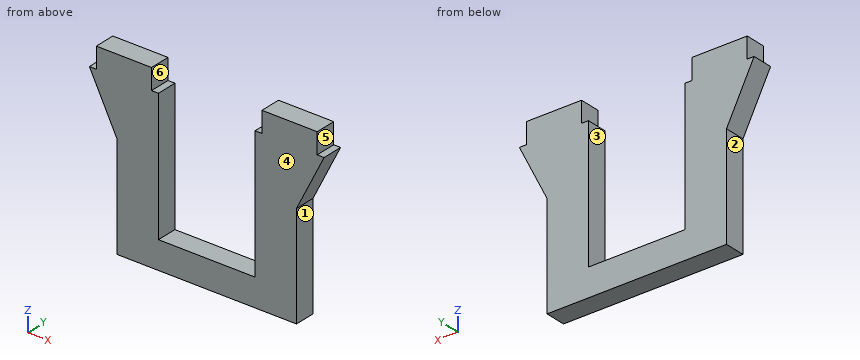
```python
from build123d import *

# Parameters (mm, degrees)
BOSS_EXTRUDE1_DEPTH = 1.5
BOSS_EXTRUDE2_DEPTH = 1.5
SKETCH3_W           = 8
SKETCH3_H           = 3
BOSS_EXTRUDE3_DEPTH = 1.5


with BuildPart() as part:
    # Sketch1 → Boss-Extrude1 (new body, symmetric)
    with BuildSketch(Plane(origin=(0, 0, 0), x_dir=(1, 0, 0), z_dir=(0, 1, 0))):
        Polygon((7, -9.5), (13, -9.5), (13, 13.5), (-13, 13.5), (-13, -9.5), (-7, -9.5), (-7, 9.5), (7, 9.5), align=None)
    extrude(amount=BOSS_EXTRUDE1_DEPTH, both=True)

    # Sketch2 → Boss-Extrude2 (add, symmetric)
    with BuildSketch(Plane(origin=(0, 0, 0), x_dir=(1, 0, 0), z_dir=(0, 1, 0))):
        Polygon((-13, -1.5), (-17, -9.5), (-13, -9.5), align=None)
        Polygon((13, -9.5), (13, -1.5), (17, -9.5), align=None)
    extrude(amount=BOSS_EXTRUDE2_DEPTH, both=True)

    # Sketch3 → Boss-Extrude3 (add, symmetric)
    with BuildSketch(Plane(origin=(0, 0, 0), x_dir=(1, 0, 0), z_dir=(0, 1, 0))):
        with Locations((-12, -11)):
            Rectangle(SKETCH3_W, SKETCH3_H)
        with Locations((12, -11)):
            Rectangle(SKETCH3_W, SKETCH3_H)
    extrude(amount=BOSS_EXTRUDE3_DEPTH, both=True)


solid = part.part
```
Could you check a few things on this model? Use its own coordinates, in mm. Face numbers are marked on the shaded views. A direction names the side the tool comes from. Coordinates: 2 decimals unless noted, no trailing zeros. Loops run counter-clockwise (first coordinate to the right, second up) from the corner with the lowest first, then second, coordinate; pieces in that order, holes last. Notation, with made-up numbers: M -1,8.5 L 36,8.5 A21 ccw 36,15.5 Z; hole C -13,88 d3. An arc over 180 degrees is marked long. Put each result on its own line as item: value. Start each with the question number.
(1) Suppose I cut it at C-C on x = 14.5. Please give me the cut outline in (y, z).
(2) For the marked faces 4, 5 and 6, which set-ups out of +Z, -Z, +X, -X, +Y, -Y let a thin tool reach every point of the face, with its end or its side?
(3) Suppose I cut it at A-A on z = 7. Please give me the cut outline in (x, y).
(4) Suppose I cut it at D-D on z = 0.5. Please give me the cut outline in (x, y).
(5) Suppose I cut it at B-B on y = 0.65. Please give me the cut outline in (x, z), then the cut area to 3 significant figures.
(6) I need wall thicknesses on line 1 (X direction, y = 0.7, z = -4); line 2 (X direction, y = -0.3, z = 7.5); line 3 (Z direction, x = -5, y = 0.9). Which ranges of each line are inside material? Lowest first, please. Write a range as from..to.
(7) Thinking about a two-plate mould opening in X: for the marked faces 1, 2 and 3, which applies, pulls with the +X half, pulls with the -X half, needs draft (parallel to the pull), parting line crosses it, or undercut?
(8) Will these pins go through, and if not, where does the flat tip stop? P1, Ø0.9, axis at y = 0, z = -5, coming from the -X side; P2, Ø1.5, axis at y = 0.5, z = 11, coming from the +X side; P3, Ø0.9, axis at x = 1, y = -0.5, coming from the +Z side.
Solutions:
1. outline: M -1.5,4.5 L 1.5,4.5 L 1.5,12.5 L -1.5,12.5 Z
2. face 4: +Z, -Z, +X, -X, -Y
2. face 5: +Z, +X, +Y, -Y
2. face 6: +Z, +Y, -Y
3. outline: M -15.75,-1.5 L -7,-1.5 L -7,1.5 L -15.75,1.5 Z; M 7,-1.5 L 15.75,-1.5 L 15.75,1.5 L 7,1.5 Z
4. outline: M -13,-1.5 L -7,-1.5 L -7,1.5 L -13,1.5 Z; M 7,-1.5 L 13,-1.5 L 13,1.5 L 7,1.5 Z
5. outline: M -17,9.5 L -13,1.5 L -13,-13.5 L 13,-13.5 L 13,1.5 L 17,9.5 L 16,9.5 L 16,12.5 L 8,12.5 L 8,9.5 L 7,9.5 L 7,-9.5 L -7,-9.5 L -7,9.5 L -8,9.5 L -8,12.5 L -16,12.5 L -16,9.5 Z
5. area: 412 mm2
6. line 1: x = -13..-7, 7..13
6. line 2: x = -16..-7, 7..16
6. line 3: z = -13.5..-9.5
7. face 1: pulls with the +X half
7. face 2: pulls with the -X half
7. face 3: undercut
8. P1: stops at x = -13
8. P2: stops at x = 16
8. P3: stops at z = -9.5
